Answer from the drawing. Dimensions are ordinates in mm from the lowest x, y and z of the part. Round coordinates to 2 decimals unless told otherwise and drop trailing zeros. Write each loop counter-clockwise with the first axis right and the second up, starting at its lowest first coordinate (ties: lowest second). Pieces come first, ordered by that corner, then holes. Notation, with made-up numbers: (-7.5, -39.5) - (39.5, -39.5) arc R32 ccw to (39.5, -7.5) - close; hole circle Ø8 at (71, 87.25). An arc over 180 degrees is marked (long way). Answer as a JSON object with one key per item and string values.
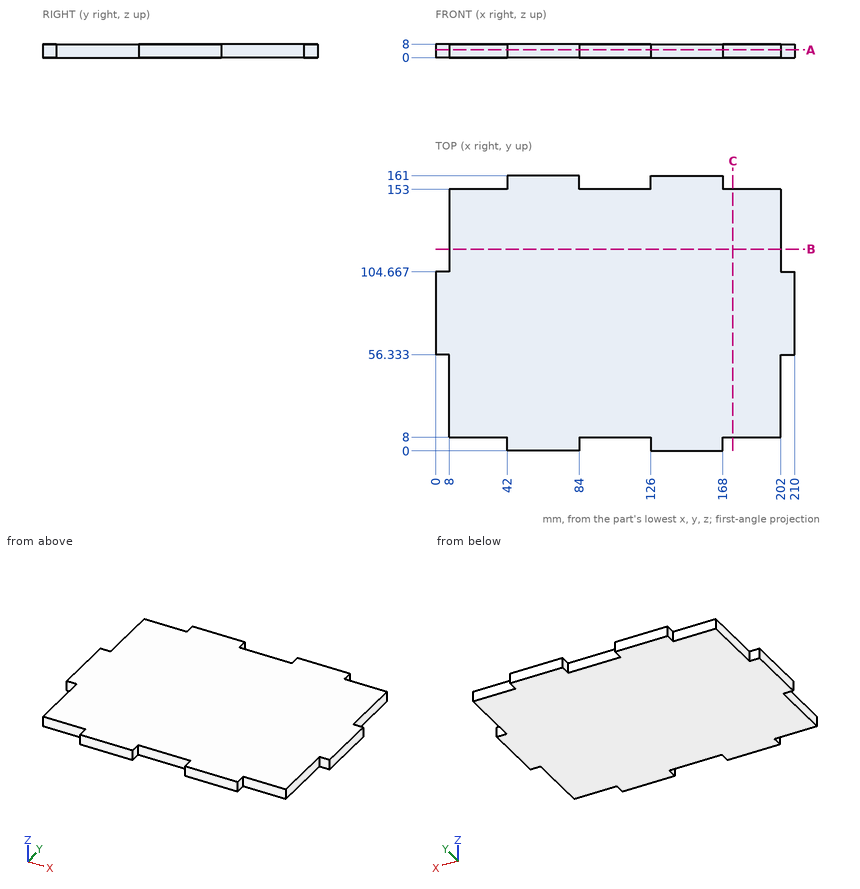
Item 1: A cutting plane is placed at A-A (z = 4.5). Write down the section's boundary in (x, y), and give its area (3 significant figures).
Results found:
{"outline": "(0, 56.33) - (8, 56.33) - (8, 8) - (42, 8) - (42, 0) - (84, 0) - (84, 8) - (126, 8) - (126, 0) - (168, 0) - (168, 8) - (202, 8) - (202, 56.33) - (210, 56.33) - (210, 104.67) - (202, 104.67) - (202, 153) - (168, 153) - (168, 161) - (126, 161) - (126, 153) - (84, 153) - (84, 161) - (42, 161) - (42, 153) - (8, 153) - (8, 104.67) - (0, 104.67) - close", "area": "30,200 mm²"}
Item 2: A cutting plane is placed at C-C (x = 174). Write down the section's boundary in (y, z).
Results found:
{"outline": "(8, 0) - (153, 0) - (153, 8) - (8, 8) - close"}
Item 3: Consider line 1 along X through (y, z) = (7, 1.5); line 2 along X through (y, z) = (137, 3.25); line 3 along Y through (x, z) = (16, 4.5). Determine where each line is inside the solid, lowest interval first.
Results found:
{"line 1": "42 to 84, 126 to 168", "line 2": "8 to 202", "line 3": "8 to 153"}
Item 4: A cutting plane is placed at B-B (y = 118). Write down the section's boundary in (x, z), and give its area (3 significant figures).
Results found:
{"outline": "(8, 0) - (202, 0) - (202, 8) - (8, 8) - close", "area": "1,550 mm²"}
Item 5: Each of these flat-tipped pins is pushed along its axis until it touches: P1, Ø1, axis at y = 37, z = 3, coming from the +X side; P2, Ø4, axis at x = 19.5, z = 5, coming from the +Y side; P3, Ø2.5, axis at x = 4, z = 5, coming from the -Y side. Where does it stop, or does it pass through?
Results found:
{"P1": "x = 202", "P2": "y = 153", "P3": "y = 56.33"}
